Check sheet for the modelled part. Datum: model origin and axes. Units: mm. Face numbers are marked on the shaded views. A direction names the side the tool comes from. Give positions to 0.01 mm unless a question says otherwise; leave off trailing zeros. Loops run counter-clockwise (first coordinate to the right, second up) from the corner with the lowest first, then second, coordinate; pieces in that order, holes last. Notation, with made-up numbers: M 15.25,-34 L 55.25,-34 A15 cw 55.25,-28 Z; hole C -6.5,-1 d4. An arc over 180 degrees is marked long. Put each result on its own line as item: value. Start each with the question number.
```python
from build123d import *

# Parameters (mm, degrees)
BOSS_EXTRUDE1_DEPTH = 2
BOSS_EXTRUDE2_DEPTH = 6
SKETCH24_R          = 3.9
BOSS_EXTRUDE5_DEPTH = 2.3
SKETCH30_W          = 2.408612022
SKETCH30_H          = 1.324178481
CUT_EXTRUDE12_DEPTH = 8
CUT_EXTRUDE11_DEPTH = 5.3
FILLET1_R           = 1.5
SKETCH34_R          = 0.75
CUT_EXTRUDE13_DEPTH = 8
SKETCH35_R          = 0.75
CUT_EXTRUDE14_DEPTH = 4
SKETCH36_R          = 0.95
CUT_EXTRUDE15_DEPTH = 8
SKETCH37_R          = 2
CUT_EXTRUDE16_DEPTH = 2.5
SKETCH38_W          = 3
SKETCH38_H          = 1.25
CUT_EXTRUDE17_DEPTH = 3.6


with BuildPart() as part:
    # Sketch2 → Boss-Extrude1 (new body)
    with BuildSketch(Plane.XY):
        with BuildLine():
            Line((-2.5, 7.5), (-16.7, 7.5))
            Line((-16.7, 7.5), (-20.7, 3.793442666))
            Line((-20.7, 3.793442666), (-20.7, -4.031648778))
            Line((-20.7, -4.031648778), (-15.7, -7.5))
            Line((-15.7, -7.5), (-6.7, -7.5))
            Line((-6.7, -7.5), (-4.2, -5.6))
            ThreePointArc((-4.2, -5.6), (3.130495168, -6.260990337), (7, 0))
            ThreePointArc((7, 0), (4.949747468, 4.949747468), (0, 7))
            Line((0, 7), (0, 7.5))
            Line((0, 7.5), (-2.5, 7.5))
        make_face()
    extrude(amount=BOSS_EXTRUDE1_DEPTH)

    # Sketch4 → Boss-Extrude2 (add)
    with BuildSketch(Plane.XY.offset(2)):
        Polygon((-15.7, -7.5), (-6.7, -7.5), (-6.759079174, -4.5), (-7.7, -4.5), (-7.7, 2), (-5.5, 2), (-5.5, 5.3), (-2.5, 5.3), (-2.5, 7.5), (-16.7, 7.5), (-20.7, 3.793442666), (-20.7, -4.031648778), align=None)
    extrude(amount=BOSS_EXTRUDE2_DEPTH)

    # Sketch24 → Boss-Extrude5 (add)
    with BuildSketch(Plane.XY.offset(2)):
        Circle(SKETCH24_R)
    extrude(amount=BOSS_EXTRUDE5_DEPTH)

    # Sketch30 → Cut-Extrude12 (cut)
    with BuildSketch(Plane(origin=(-5.5, 0, 0), x_dir=(0, 0, -1), z_dir=(1, 0, 0))):
        with Locations((-3.261593395, 4.63791076)):
            Rectangle(SKETCH30_W, SKETCH30_H)
    extrude(amount=-CUT_EXTRUDE12_DEPTH, mode=Mode.SUBTRACT)

    # Sketch28 → Cut-Extrude11 (cut, through all)
    with BuildSketch(Plane.XY.offset(4.3)):
        with BuildLine():
            Line((-1, 1.732050808), (-1, -1.732050808))
            ThreePointArc((-1, -1.732050808), (2, 0), (-1, 1.732050808))
        make_face()
    extrude(amount=-CUT_EXTRUDE11_DEPTH, mode=Mode.SUBTRACT)

    # Fillet1
    fillet1_edges = [part.edges().sort_by_distance(p)[0] for p in [
        (-11.2, -7.5, 0),
        (-8.35, 7.5, 0),
        (-18.7, 5.646721333, 0),
        (-18.2, -5.765824389, 0),
        (-20.7, -0.119103056, 0),
        (-15.7, -7.5, 4),
        (-20.7, -4.031648778, 4),
        (-20.7, 3.793442666, 4),
        (-16.7, 7.5, 4),
    ]]
    fillet(fillet1_edges, radius=FILLET1_R)

    # Sketch34 → Cut-Extrude13 (cut, along a direction that is not the sketch's normal)
    with BuildSketch(Plane.XZ.offset(-2)):
        with Locations((-7, 8)):
            Circle(SKETCH34_R)
    extrude(amount=-CUT_EXTRUDE13_DEPTH, dir=(0.668583388, -0.743637179, 0), mode=Mode.SUBTRACT)

    # Sketch35 → Cut-Extrude14 (cut, symmetric, along a direction that is not the sketch's normal)
    with BuildSketch(Plane(origin=(0, -4.5, 0), x_dir=(1, 0, 0), z_dir=(0, 1, 0))):
        with Locations((-8.259079174, -8)):
            Circle(SKETCH35_R)
    extrude(amount=CUT_EXTRUDE14_DEPTH, dir=(0.599919418, 0.80006043, 0), both=True, mode=Mode.SUBTRACT)

    # Sketch36 → Cut-Extrude15 (cut)
    with BuildSketch(Plane.XY.offset(8)):
        with Locations((-11.7, 0)):
            Circle(SKETCH36_R)
        with Locations((-16.7, 0)):
            Circle(SKETCH36_R)
    extrude(amount=-CUT_EXTRUDE15_DEPTH, mode=Mode.SUBTRACT)

    # Sketch37 → Cut-Extrude16 (cut)
    with BuildSketch(Plane(origin=(0, 0, 0), x_dir=(-1, 0, 0), z_dir=(0, 0, -1))):
        with Locations((11.7, 0)):
            Circle(SKETCH37_R)
        with Locations((16.7, 0)):
            Circle(SKETCH37_R)
    extrude(amount=-CUT_EXTRUDE16_DEPTH, mode=Mode.SUBTRACT)

    # Sketch38 → Cut-Extrude17 (cut)
    with BuildSketch(Plane.XY.offset(8)):
        with Locations((-4, 5.925)):
            Rectangle(SKETCH38_W, SKETCH38_H)
    extrude(amount=-CUT_EXTRUDE17_DEPTH, mode=Mode.SUBTRACT)

    # Mirror1: part across plane


with BuildPart() as part_1:
    add(part.part)
    add(part.part.mirror(Plane.XY.offset(8)))


with BuildPart() as body_2:
    # Split1: the piece on the far side of the plane
    add(part_1.part)
    split(bisect_by=Plane.XY.offset(8), keep=Keep.BOTTOM)


with BuildPart() as part_2:
    add(part_1.part)

    # Split1
    split(bisect_by=Plane.XY.offset(8), keep=Keep.TOP)


solid = part_2.part
```
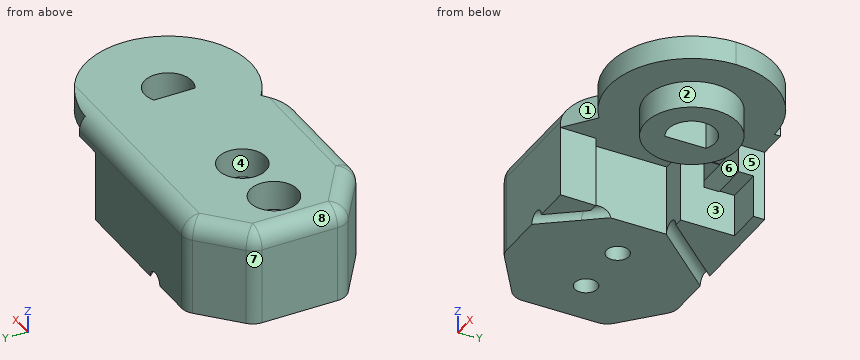
Q1. Access from +Z, -Z, +X, -X, +Y, -Y to the whole of each face (thin tool, end or side, straight path). Record for the marked faces 1, 2, 3, 4 and 5.
Q2. Mould release check, pull along Y, two halves, no side actions. Record for the marked faces 6, 7 and 8: pulls with the +Y half, pulls with the -Y half, needs draft (parallel to the pull), parting line crosses it, or undercut.
Q3. Section check B-B, the plane x = -11.7. Give the number of separate pieces and of enclosed holes in the cut face, then the cut area to 3 significant figures.
Q4. Depth check by flat-ended pin: P1, Ø1, axis at y = -3, z = 9, coming from the +X side; P2, Ø3, axis at x = 4, z = 13.5, coming from the +Y side; P3, Ø0.7, axis at y = 6, z = 11.5, coming from the +X side. Enter the tip coordinate at first touch or a pass-through.
Q5. Thickness scan on line 1 along Y through (x, z) = (-11.7, 12.3); line 2 along Y through (x, z) = (-11.7, 9.8); line 3 along Z through (x, y) = (-1.5, 5.25). Record the ranges inside material, lowest first. Write a range as [from, to].
Q6. Section check A-A, the plane z = 10.75. Record the cut outline in (x, y), then the cut area to 3 significant figures.
Found:
1. face 1: +Z, -Z, -Y
1. face 2: -Z
1. face 3: -Z, -Y
1. face 4: +Z
1. face 5: -Z, +X, +Y
2. face 6: undercut
2. face 7: pulls with the +Y half
2. face 8: needs draft
3. separate pieces: 2
3. enclosed holes: 1
3. area: 94.7 mm^2
4. P1: stops at x = -7.7
4. P2: stops at y = 6.5
4. P3: stops at x = -2.5
5. line 1: y = [-7.5, -0.95], [0.95, 3.98], [5.3, 7.5]
5. line 2: y = [-7.5, -0.95], [0.95, 7.5]
5. line 3: z = [14, 16]
6. outline: M -20.7,-3.25 A1.5 ccw -20.05,-4.48 L -16.09,-7.23 A1.5 ccw -15.23,-7.5 L -6.7,-7.5 L -6.76,-4.5 L -7.7,-4.5 L -7.7,2 L -5.5,2 L -5.5,6.55 L -2.5,6.55 L -2.5,7.5 L -16.11,7.5 A1.5 ccw -17.13,7.1 L -20.22,4.24 A1.5 ccw -20.7,3.14 Z; hole C -16.7,0 d1.9; hole C -11.7,0 d1.9
6. area: 191 mm^2
